Autodesk Inventor part; units mm, degrees
ref_plane "YZ Plane" through (0, 0, 0) normal (1, 0, 0) x (0, 1, 0)
ref_plane "XZ Plane" through (0, 0, 0) normal (0, 1, 0) x (-1, 0, 0)
ref_plane "XY Plane" through (0, 0, 0) normal (0, 0, 1) x (1, 0, 0)
sketch "Sketch1" plane through (0, 0, 0) normal (0, 1, 0) x (-1, 0, 0)
  line L0 (0, 0) -> (-15, 0)
  line L1 (-15, 0) -> (-15, 27.3)
  line L2 (-15, 27.3) -> (0, 27.3)
  line L3 (0, 27.3) -> (0, 0)
  line L4 (-3, 0) -> (-3, 27.3)
  line L5 (-5.5, 0) -> (-5.5, 27.3)
  line L6 (0, 2) -> (-3, 2)
  line L7 (0, 25.3) -> (-3, 25.3)
  line L8 (-5.5, 2) -> (-15, 2)
  line L9 (-5.5, 25.3) -> (-15, 25.3)
  dimension "d0" = 27.3
  dimension "d1" = 15
  dimension "d2" = 3
  dimension "d3" = 2.5
  dimension "d4" = 2
  dimension "d5" = 2
  dimension "d6" = 2
  dimension "d7" = 2
extrude "Extrusion1" add sketch "Sketch1" against normal blind 2
extrude "Extrusion2" add sketch "Sketch1" along normal blind 14.2 contours L0 L4 L6 L3 | L0 L1 L8 L5 | L7 L4 L2 L3 | L9 L1 L2 L5
sketch "Sketch2" plane through (15, -2, 27.3) normal (1, 0, 0) x (0, 0, -1)
  line L0 (25.3, 2) -> (25.3, 16.2)
  line L1 (2, 2) -> (2, 16.2)
  line L2 (25.3, 16.2) -> (27.3, 16.2)
  line L3 (2, 16.2) -> (2.8, 14.2)
  line L4 (2.8, 14.2) -> (2, 14.2)
  line L5 (25.3, 16.2) -> (24.5, 14.2)
  line L6 (24.5, 14.2) -> (25.3, 14.2)
  point P0 (27.3, 2)
  dimension "d12" = 2
  dimension "d13" = 2
  dimension "d14" = 0.8
  dimension "d15" = 0.8
extrude "Extrusion3" add sketch "Sketch2" against normal up to surface (15 mm away)
sketch "Sketch3" plane through (0, -2, 27.3) normal (0, 0, 1) x (1, 0, 0)
  line L0 (3, 14.2) -> (3, 16.2)
  line L1 (5.5, 14.2) -> (3, 14.2)
  line L2 (5.5, 14.2) -> (5.5, 16.2)
  line L3 (5.5, 16.2) -> (3, 16.2)
  point P0 (0, 2)
extrude "Extrusion4" cut sketch "Sketch3" against normal through all
properties part number "servo clip"
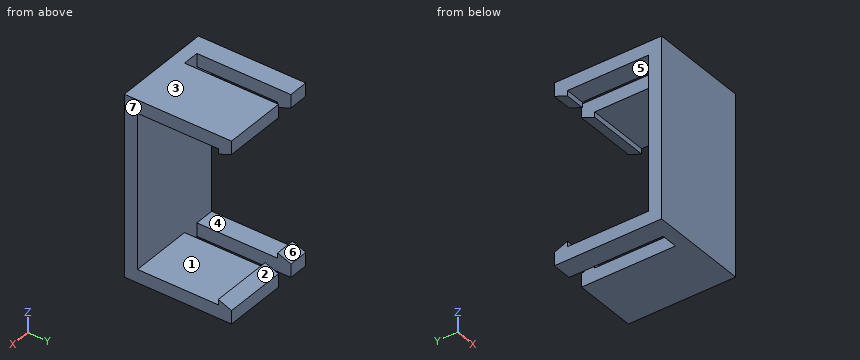
Verification items for the finished model (mm, model axes). Face numbers are marked on the shaded views. A direction names the side the tool comes from. Round coordinates to 2 decimals unless told otherwise and drop trailing zeros. Order: outer loops, then holes, each group sorted by start corner. A loop starts at its lowest first (then second) coordinate and runs counter-clockwise, first axis right, second up.
1. Access from +Z, -Z, +X, -X, +Y, -Y to the whole of each face (thin tool, end or side, straight path). Record for the marked faces 1, 2 and 3.
Final values:
face 1: +X, -X
face 2: +X, -X, +Y
face 3: +Z, +X, -X, +Y, -Y
2. Release check for a two-part mould opening along Y. For the marked faces 4, 5, 6 and 7 record: +Y half, -Y half, draft (parallel to the pull), parting line (faces both ways), or undercut.
Final values:
face 4: undercut
face 5: undercut
face 6: +Y half
face 7: draft
3. Section check A-A on y = 13.25. Record the cut outline in (x, z), then the cut area to 3 significant figures.
Final values:
outline: (0, 0) - (3, 0) - (3, 2.38) - (0, 2.38) - close; (0, 24.92) - (3, 24.92) - (3, 27.3) - (0, 27.3) - close; (5.5, 0) - (15, 0) - (15, 2.38) - (5.5, 2.38) - close; (5.5, 24.92) - (15, 24.92) - (15, 27.3) - (5.5, 27.3) - close
area: 59.5 mm2
4. Section check D-D on y = 11.5. Record the cut outline in (x, z).
Final values:
outline: (0, 0) - (3, 0) - (3, 2) - (0, 2) - close; (0, 25.3) - (3, 25.3) - (3, 27.3) - (0, 27.3) - close; (5.5, 0) - (15, 0) - (15, 2) - (5.5, 2) - close; (5.5, 25.3) - (15, 25.3) - (15, 27.3) - (5.5, 27.3) - close
5. Go/stop test with a flat-tipped pin: P1, Ø6, axis at x = 9, z = 6.5, coming from the +Y side. Record where the tip stops, or that it passes through.
Final values:
P1: stops at y = 0
6. Section check C-C on x = 7. Record the cut outline in (y, z), then the cut area to 3 significant figures.
Final values:
outline: (-2, 0) - (14.2, 0) - (14.2, 2) - (12.2, 2.8) - (12.2, 2) - (0, 2) - (0, 25.3) - (12.2, 25.3) - (12.2, 24.5) - (14.2, 25.3) - (14.2, 27.3) - (-2, 27.3) - close
area: 113 mm2
7. Thickness scan on L1, parallel to Z at x = 14.5, y = 6; L2, parallel to Y at x = 8.25, z = 22.75; L3, parallel to Z at x = 9, y = 12.5. Record the ranges inside material, lowest first.
Final values:
L1: z = 0 to 2, 25.3 to 27.3
L2: y = -2 to 0
L3: z = 0 to 2.68, 24.62 to 27.3
8. Section check B-B on z = 25. Record the cut outline in (x, y).
Final values:
outline: (0, -2) - (15, -2) - (15, 0) - (0, 0) - close; (0, 12.2) - (3, 12.2) - (3, 13.45) - (0, 13.45) - close; (5.5, 12.2) - (15, 12.2) - (15, 13.45) - (5.5, 13.45) - close
